Can you work these out from the model? Positions are in its coordinate system, mm. Face numbers are marked on the shaded views. A direction names the side the tool comes from. Coordinates: 2 decimals unless noted, no trailing zeros. Loops run counter-clockwise (first coordinate to the right, second up) from the corner with the lowest first, then second, coordinate; pieces in that order, holes last.
```python
from build123d import *

# Parameters (mm, degrees)
BOSS_EXTRUDE1_DEPTH     = 1.27
FILLET1_R               = 2
BOSS_EXTRUDE2_DEPTH     = 4
CUT_EXTRUDE1_DEPTH      = 49.880756713
CUT_EXTRUDE1_DEPTH_BACK = 49.880756713
SKETCH3_R               = 2.5
FILLET2_R               = 2


with BuildPart() as part:
    # Sketch1 → Boss-Extrude1 (new, symmetric)
    with BuildSketch(Plane.XY):
        Polygon((-45, 0), (-20, 8), (20, 8), (45, 0), (20, -8), (-20, -8), align=None)
    extrude(amount=BOSS_EXTRUDE1_DEPTH, both=True)

    # Fillet1
    fillet1_edges = [part.edges().sort_by_distance(p)[0] for p in [
        (-45, 0, 0),
        (45, 0, 0),
    ]]
    fillet(fillet1_edges, radius=FILLET1_R)

    # Sketch2 → Boss-Extrude2 (add, symmetric)
    with BuildSketch(Plane(origin=(0, 0, 0), x_dir=(1, 0, 0), z_dir=(0, 1, 0))):
        Polygon((-32.437797626, 1.27), (-32.437797626, 26.27), (-19.437797626, 26.27), (-19.437797626, 16.27), (-22.437797626, 16.27), (-22.437797626, 1.27), align=None)
        Polygon((22.437797626, 16.27), (22.437797626, 1.27), (32.437797626, 1.27), (32.437797626, 26.27), (19.437797626, 26.27), (19.437797626, 16.27), align=None)
    extrude(amount=BOSS_EXTRUDE2_DEPTH, both=True)

    # Sketch3 → Cut-Extrude1 (cut, two sides: drawn at the far end of the back side and taken through both)
    with BuildSketch(Plane(origin=(0, 0, 0), x_dir=(0, 0, -1), z_dir=(1, 0, 0)).offset(-CUT_EXTRUDE1_DEPTH_BACK)):
        with Locations((22.350351111, 0)):
            Circle(SKETCH3_R)
    extrude(amount=CUT_EXTRUDE1_DEPTH + CUT_EXTRUDE1_DEPTH_BACK, mode=Mode.SUBTRACT)

    # Fillet2
    # the kernel refuses this fillet: 2 mm, written as the material it adds along each edge
    with BuildSketch(Plane(origin=(-22.437797626, -4, -1.27), x_dir=(0, -1, 0), z_dir=(-1, 0, 0))) as fillet2_piece_1_section:
        with BuildLine():
            CenterArc((FILLET2_R, -FILLET2_R), FILLET2_R, 90, 90)
            Line((0, -FILLET2_R), (0, 0))
            Line((0, 0), (FILLET2_R, 0))
        make_face()
    fillet2_piece_1 = extrude(amount=10, mode=Mode.PRIVATE)
    fillet2_piece_1 = split(fillet2_piece_1, bisect_by=Plane(origin=(-27.271019309, -5.673273821, -1.76186219), z_dir=(0.3047757271037839, 0.9524241471993241, 0)), keep=Keep.TOP, mode=Mode.PRIVATE)
    add(fillet2_piece_1)
    with BuildSketch(Plane(origin=(-22.437797626, -4, -1.27), x_dir=(1, 0, 0), z_dir=(0, 1, 0))) as fillet2_piece_2:
        with BuildLine():
            CenterArc((FILLET2_R, FILLET2_R), FILLET2_R, 180, 90)
            Line((0, FILLET2_R), (0, 0))
            Line((0, 0), (FILLET2_R, 0))
        make_face()
    extrude(amount=8)
    with BuildSketch(Plane(origin=(-22.437797626, 4, -1.27), x_dir=(0, 1, 0), z_dir=(-1, 0, 0))) as fillet2_piece_3_section:
        with BuildLine():
            CenterArc((FILLET2_R, FILLET2_R), FILLET2_R, 180, 90)
            Line((0, FILLET2_R), (0, 0))
            Line((0, 0), (FILLET2_R, 0))
        make_face()
    fillet2_piece_3 = extrude(amount=10, mode=Mode.PRIVATE)
    fillet2_piece_3 = split(fillet2_piece_3, bisect_by=Plane(origin=(-27.271019309, 5.673273821, -1.76186219), z_dir=(0.3047757271037837, -0.9524241471993242, 0)), keep=Keep.TOP, mode=Mode.PRIVATE)
    add(fillet2_piece_3)
    with BuildSketch(Plane(origin=(22.437797626, -4, -1.27), x_dir=(0, -1, 0), z_dir=(1, 0, 0))) as fillet2_piece_4_section:
        with BuildLine():
            CenterArc((FILLET2_R, FILLET2_R), FILLET2_R, 180, 90)
            Line((0, FILLET2_R), (0, 0))
            Line((0, 0), (FILLET2_R, 0))
        make_face()
    fillet2_piece_4 = extrude(amount=10, mode=Mode.PRIVATE)
    fillet2_piece_4 = split(fillet2_piece_4, bisect_by=Plane(origin=(27.271019309, -5.673273821, -1.76186219), z_dir=(-0.30477572710378414, 0.9524241471993241, 0)), keep=Keep.TOP, mode=Mode.PRIVATE)
    add(fillet2_piece_4)
    with BuildSketch(Plane(origin=(22.437797626, -4, -1.27), x_dir=(-1, 0, 0), z_dir=(0, 1, 0))) as fillet2_piece_5:
        with BuildLine():
            CenterArc((FILLET2_R, -FILLET2_R), FILLET2_R, 90, 90)
            Line((0, -FILLET2_R), (0, 0))
            Line((0, 0), (FILLET2_R, 0))
        make_face()
    extrude(amount=8)
    with BuildSketch(Plane(origin=(22.437797626, 4, -1.27), x_dir=(0, 1, 0), z_dir=(1, 0, 0))) as fillet2_piece_6_section:
        with BuildLine():
            CenterArc((FILLET2_R, -FILLET2_R), FILLET2_R, 90, 90)
            Line((0, -FILLET2_R), (0, 0))
            Line((0, 0), (FILLET2_R, 0))
        make_face()
    fillet2_piece_6 = extrude(amount=10, mode=Mode.PRIVATE)
    fillet2_piece_6 = split(fillet2_piece_6, bisect_by=Plane(origin=(27.271019309, 5.673273821, -1.76186219), z_dir=(-0.30477572710378353, -0.9524241471993244, 0)), keep=Keep.TOP, mode=Mode.PRIVATE)
    add(fillet2_piece_6)
    with BuildSketch(Plane(origin=(-22.437797626, -9, -1.27), x_dir=(1, 0, 0), z_dir=(0, 1, 0))) as fillet2_piece_7a_section:
        with BuildLine():
            CenterArc((FILLET2_R, FILLET2_R), FILLET2_R, 180, 90)
            Line((0, FILLET2_R), (0, 0))
            Line((0, 0), (FILLET2_R, 0))
        make_face()
    fillet2_piece_7a = extrude(amount=13, mode=Mode.PRIVATE)
    fillet2_piece_7a = split(fillet2_piece_7a, bisect_by=Plane(origin=(-22.456507994, -7.213917442, -1.712345443), z_dir=(0.3047757271037839, 0.9524241471993241, 0)), keep=Keep.TOP, mode=Mode.PRIVATE)
    fillet2_piece_7a = split(fillet2_piece_7a, bisect_by=Plane(origin=(-21.967327257, -4, -1.712345443), z_dir=(0, -1, 0)), keep=Keep.TOP, mode=Mode.PRIVATE)
    with BuildSketch(Plane(origin=(-17.437797626, -4, -1.27), x_dir=(0, -1, 0), z_dir=(-1, 0, 0))) as fillet2_piece_7b_section:
        with BuildLine():
            CenterArc((FILLET2_R, -FILLET2_R), FILLET2_R, 90, 90)
            Line((0, -FILLET2_R), (0, 0))
            Line((0, 0), (FILLET2_R, 0))
        make_face()
    fillet2_piece_7b = extrude(amount=15, mode=Mode.PRIVATE)
    fillet2_piece_7b = split(fillet2_piece_7b, bisect_by=Plane(origin=(-22.437797626, -4.452790229, -1.722790229), z_dir=(1, 0, 0)), keep=Keep.TOP, mode=Mode.PRIVATE)
    fillet2_piece_7 = fillet2_piece_7a & fillet2_piece_7b
    add(fillet2_piece_7)
    with BuildSketch(Plane(origin=(-17.437797626, 4, -1.27), x_dir=(0, 1, 0), z_dir=(-1, 0, 0))) as fillet2_piece_8a_section:
        with BuildLine():
            CenterArc((FILLET2_R, FILLET2_R), FILLET2_R, 180, 90)
            Line((0, FILLET2_R), (0, 0))
            Line((0, 0), (FILLET2_R, 0))
        make_face()
    fillet2_piece_8a = extrude(amount=15, mode=Mode.PRIVATE)
    fillet2_piece_8a = split(fillet2_piece_8a, bisect_by=Plane(origin=(-22.437797626, 4.452790229, -1.722790229), z_dir=(1, 0, 0)), keep=Keep.TOP, mode=Mode.PRIVATE)
    with BuildSketch(Plane(origin=(-22.437797626, -4, -1.27), x_dir=(1, 0, 0), z_dir=(0, 1, 0))) as fillet2_piece_8b_section:
        with BuildLine():
            CenterArc((FILLET2_R, FILLET2_R), FILLET2_R, 180, 90)
            Line((0, FILLET2_R), (0, 0))
            Line((0, 0), (FILLET2_R, 0))
        make_face()
    fillet2_piece_8b = extrude(amount=13, mode=Mode.PRIVATE)
    fillet2_piece_8b = split(fillet2_piece_8b, bisect_by=Plane(origin=(-22.456507994, 7.213917442, -1.712345443), z_dir=(0.3047757271037837, -0.9524241471993242, 0)), keep=Keep.TOP, mode=Mode.PRIVATE)
    fillet2_piece_8b = split(fillet2_piece_8b, bisect_by=Plane(origin=(-21.967327257, 4, -1.712345443), z_dir=(0, 1, 0)), keep=Keep.TOP, mode=Mode.PRIVATE)
    fillet2_piece_8 = fillet2_piece_8a & fillet2_piece_8b
    add(fillet2_piece_8)
    with BuildSketch(Plane(origin=(22.437797626, -9, -1.27), x_dir=(-1, 0, 0), z_dir=(0, 1, 0))) as fillet2_piece_9a_section:
        with BuildLine():
            CenterArc((FILLET2_R, -FILLET2_R), FILLET2_R, 90, 90)
            Line((0, -FILLET2_R), (0, 0))
            Line((0, 0), (FILLET2_R, 0))
        make_face()
    fillet2_piece_9a = extrude(amount=13, mode=Mode.PRIVATE)
    fillet2_piece_9a = split(fillet2_piece_9a, bisect_by=Plane(origin=(22.456507994, -7.213917442, -1.712345443), z_dir=(-0.30477572710378414, 0.9524241471993241, 0)), keep=Keep.TOP, mode=Mode.PRIVATE)
    fillet2_piece_9a = split(fillet2_piece_9a, bisect_by=Plane(origin=(21.967327257, -4, -1.712345443), z_dir=(0, -1, 0)), keep=Keep.TOP, mode=Mode.PRIVATE)
    with BuildSketch(Plane(origin=(17.437797626, -4, -1.27), x_dir=(0, -1, 0), z_dir=(1, 0, 0))) as fillet2_piece_9b_section:
        with BuildLine():
            CenterArc((FILLET2_R, FILLET2_R), FILLET2_R, 180, 90)
            Line((0, FILLET2_R), (0, 0))
            Line((0, 0), (FILLET2_R, 0))
        make_face()
    fillet2_piece_9b = extrude(amount=15, mode=Mode.PRIVATE)
    fillet2_piece_9b = split(fillet2_piece_9b, bisect_by=Plane(origin=(22.437797626, -4.452790229, -1.722790229), z_dir=(-1, 0, 0)), keep=Keep.TOP, mode=Mode.PRIVATE)
    fillet2_piece_9 = fillet2_piece_9a & fillet2_piece_9b
    add(fillet2_piece_9)
    with BuildSketch(Plane(origin=(22.437797626, -4, -1.27), x_dir=(-1, 0, 0), z_dir=(0, 1, 0))) as fillet2_piece_10a_section:
        with BuildLine():
            CenterArc((FILLET2_R, -FILLET2_R), FILLET2_R, 90, 90)
            Line((0, -FILLET2_R), (0, 0))
            Line((0, 0), (FILLET2_R, 0))
        make_face()
    fillet2_piece_10a = extrude(amount=13, mode=Mode.PRIVATE)
    fillet2_piece_10a = split(fillet2_piece_10a, bisect_by=Plane(origin=(22.456507994, 7.213917442, -1.712345443), z_dir=(-0.30477572710378353, -0.9524241471993244, 0)), keep=Keep.TOP, mode=Mode.PRIVATE)
    fillet2_piece_10a = split(fillet2_piece_10a, bisect_by=Plane(origin=(21.967327257, 4, -1.712345443), z_dir=(0, 1, 0)), keep=Keep.TOP, mode=Mode.PRIVATE)
    with BuildSketch(Plane(origin=(17.437797626, 4, -1.27), x_dir=(0, 1, 0), z_dir=(1, 0, 0))) as fillet2_piece_10b_section:
        with BuildLine():
            CenterArc((FILLET2_R, -FILLET2_R), FILLET2_R, 90, 90)
            Line((0, -FILLET2_R), (0, 0))
            Line((0, 0), (FILLET2_R, 0))
        make_face()
    fillet2_piece_10b = extrude(amount=15, mode=Mode.PRIVATE)
    fillet2_piece_10b = split(fillet2_piece_10b, bisect_by=Plane(origin=(22.437797626, 4.452790229, -1.722790229), z_dir=(-1, 0, 0)), keep=Keep.TOP, mode=Mode.PRIVATE)
    fillet2_piece_10 = fillet2_piece_10a & fillet2_piece_10b
    add(fillet2_piece_10)


solid = part.part
```
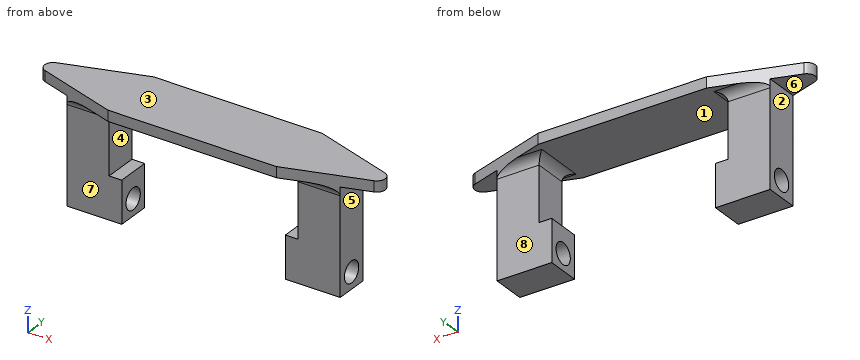
Item 1: Suppose I cut it at B-B, the plane y = 0. Please give me the cut outline in (x, z), plus the area to 3 significant figures.
Results are:
outline: (-40.44, -1.27) - (-32.44, -1.27) - (-32.44, -19.85) - (-19.44, -19.85) - (-19.44, -16.27) - (-22.44, -16.27) - (-22.44, -3.27) arc R2 cw to (-20.44, -1.27) - (20.44, -1.27) arc R2 cw to (22.44, -3.27) - (22.44, -16.27) - (19.44, -16.27) - (19.44, -19.85) - (32.44, -19.85) - (32.44, -1.27) - (40.44, -1.27) - (40.44, 1.27) - (-40.44, 1.27) - close; (-32.44, -26.27) - (-19.44, -26.27) - (-19.44, -24.85) - (-32.44, -24.85) - close; (19.44, -26.27) - (32.44, -26.27) - (32.44, -24.85) - (19.44, -24.85) - close
area: 637 mm2
Item 2: I need wall thicknesses on line 1 along X through (y, z) = (1.25, -20); line 2 along Z through (x, y) = (29, 0.25); line 3 along Z through (x, y) = (28.75, 0). Which ranges of each line are inside material? Lowest first, please.
Results are:
line 1: x = -32.44 to -19.44, 19.44 to 32.44
line 2: z = -26.27 to -24.84, -19.86 to 1.27
line 3: z = -26.27 to -24.85, -19.85 to 1.27
Item 3: On a 3-axis mill with a long thin cutter (end or side, diameter ignored), from which of +Z, -Z, +X, -X, +Y, -Y can I reach the whole of each face in a straight line? I mean the marked faces 5, 6, 7 and 8. Say none if no direction works.
Results are:
face 5: -Z, +X, +Y, -Y
face 6: -Z, -X, +Y, -Y
face 7: -Z, +X, -X, -Y
face 8: -Z, +X, -X, +Y
Item 4: Suppose I cut it at C-C, the plane x = 7. Please give me the cut outline in (y, z).
Results are:
outline: (-8, -1.27) - (8, -1.27) - (8, 1.27) - (-8, 1.27) - close
Item 5: Suppose I cut it at A-A, the plane z = -12. Please give me the cut outline in (x, y), plus the area to 3 significant figures.
Results are:
outline: (-32.44, -4) - (-22.44, -4) - (-22.44, 4) - (-32.44, 4) - close; (22.44, -4) - (32.44, -4) - (32.44, 4) - (22.44, 4) - close
area: 160 mm2
Item 6: We'd pull the mould along X, two halves only. Please class the marked faces 1, 2, 3 and 4: +X half, -X half, draft (parallel to the pull), parting line (faces both ways), or undercut.
Results are:
face 1: undercut
face 2: -X half
face 3: draft
face 4: undercut
Item 7: I'm going to push flat-ended pins straight in: P1, Ø4, axis at x = 24.5, z = -12, coming from the +Y side; P2, Ø10.5, axis at x = -25.5, z = -16, coming from the -Y side; P3, Ø9, axis at y = 0, z = -6.5, coming from the -X side; P4, Ø9, axis at x = 35, y = -1.5, coming from the -Z side. Where does each tip first touch, or does it pass through?
Results are:
P1: stops at y = 4
P2: stops at y = -4
P3: stops at x = -32.44
P4: stops at z = -26.27
